For this review, take the finished solid that the model builds, in its own axes (mm). Face numbers are marked on the shaded views. A direction names the side the tool comes from. Round coordinates to 2 decimals unless told otherwise and drop trailing zeros. Order: outer loops, then holes, each group sorted by start corner. A loop starts at its lowest first (then second) coordinate and runs counter-clockwise, first axis right, second up. Notation, with made-up numbers: M -20,-14 L -12,-14 A15 cw -12,3 Z; hole C -15,-13 d6. An arc over 180 degrees is marked long. Answer in a Markdown table with one row per item. Add a question column.
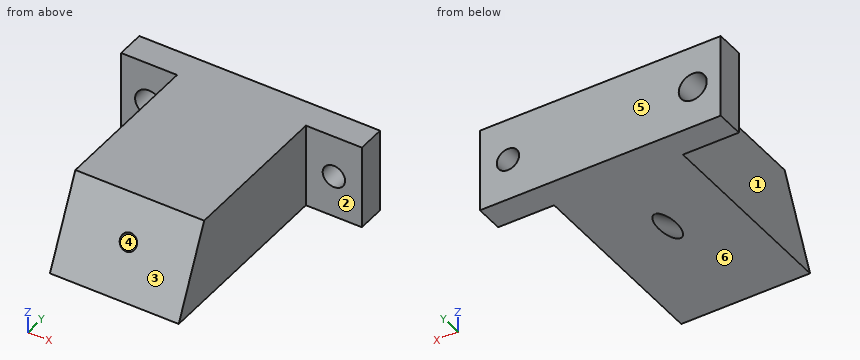
```python
from build123d import *

# Parameters (mm, degrees)
SKETCH1_W           = 23
SKETCH1_H           = 15
BOSS_EXTRUDE1_DEPTH = 40
CUT_EXTRUDE1_DEPTH  = 40
SKETCH3_R           = 1.5
CUT_EXTRUDE2_DEPTH  = 36
SKETCH4_W           = 15
SKETCH4_H           = 5
BOSS_EXTRUDE2_DEPTH = 10
SKETCH5_W           = 15
SKETCH5_H           = 5
BOSS_EXTRUDE3_DEPTH = 10
SKETCH6_R           = 2.5
SKETCH6_R_2         = 2
CUT_EXTRUDE3_DEPTH  = 10


with BuildPart() as part:
    # Sketch1 → Boss-Extrude1 (new body)
    with BuildSketch(Plane(origin=(0, 0, 0), x_dir=(1, 0, 0), z_dir=(0, 1, 0))):
        with Locations((-65.404761905, 8.571428571)):
            Rectangle(SKETCH1_W, SKETCH1_H)
    extrude(amount=BOSS_EXTRUDE1_DEPTH)

    # Sketch2 → Cut-Extrude1 (cut)
    with BuildSketch(Plane(origin=(-53.904761905, 0, 0), x_dir=(0, 0, -1), z_dir=(1, 0, 0))):
        Polygon((16.071428571, 0), (1.071428571, 0), (1.071428571, 6.994614872), align=None)
    extrude(amount=-CUT_EXTRUDE1_DEPTH, mode=Mode.SUBTRACT)

    # Sketch3 → Cut-Extrude2 (cut)
    with BuildSketch(Plane(origin=(0, 6.155714275, -2.870456708), x_dir=(1, 0, 0), z_dir=(0, -0.9063077870366528, 0.4226182617406934))):
        with Locations(Location((-65.378595466, -5.514992079, 0), (0, 0, 270))):
            Circle(SKETCH3_R)
    extrude(amount=-CUT_EXTRUDE2_DEPTH, mode=Mode.SUBTRACT)

    # Sketch4 → Boss-Extrude2 (add)
    with BuildSketch(Plane(origin=(-53.904761905, 0, 0), x_dir=(0, 0, -1), z_dir=(1, 0, 0))):
        with Locations((8.571428571, 37.5)):
            Rectangle(SKETCH4_W, SKETCH4_H)
    extrude(amount=BOSS_EXTRUDE2_DEPTH)

    # Sketch5 → Boss-Extrude3 (add)
    with BuildSketch(Plane.ZY.offset(76.904761905)):
        with Locations((-8.571428571, 37.5)):
            Rectangle(SKETCH5_W, SKETCH5_H)
    extrude(amount=BOSS_EXTRUDE3_DEPTH)

    # Sketch6 → Cut-Extrude3 (cut)
    with BuildSketch(Plane.XZ.offset(-35)):
        with Locations(Location((-81.904761905, -8.571428571, 0), (0, 0, 270))):
            Circle(SKETCH6_R)
        with Locations(Location((-48.904761905, -8.571428571, 0), (0, 0, 270))):
            Circle(SKETCH6_R_2)
    extrude(amount=-CUT_EXTRUDE3_DEPTH, mode=Mode.SUBTRACT)


solid = part.part
```
1. Consider section D-D on y = 30. Write out the cut boundary in (x, z), plus the area to 3 significant figures.
2. For the marked faces 1, 2 and 3, list the 3-axis set-ups (+Z, -Z, +X, -X, +Y, -Y) from which the entire face can be reached by the end or side of a thin tool; tool diameter is ignored.
3. Consider section B-B on x = -72. Write out the cut boundary in (y, z).
4. To check wall thickness, follow probe 1 along Y at (x, z) = (-83, -11); probe 2 along X at (y, z) = (20.5, -11); probe 3 along X at (y, z) = (7, -10.25). State the ranges of each line that lie inside material, in increasing order. Write a range as [from, to].
5. Consider section A-A on z = -9.75. State how many separate pieces and enclosed holes the cut face has, plus the area to 3 significant figures.
6. The part is to be moulded in two halves that separate along Y. For the marked faces 4, 5 and 6, say which applies: pulls with the +Y half, pulls with the -Y half, needs draft (parallel to the pull), parting line crosses it, or undercut.
7. Clearance check with flat-ended pins moving along their axes: pin 1 Ø2 at (y, z) = (6, -8.5) entering from -X; pin 2 Ø5 at (y, z) = (26.5, -6) entering from +X; pin 3 Ø8 at (x, z) = (-51.5, -7) entering from -Y. State where each tip first meets the part, or that it passes through.
Solved:
| question | item | result |
|---|---|---|
| 1 | outline | M -76.9,-16.07 L -53.9,-16.07 L -53.9,-1.07 L -76.9,-1.07 Z |
| 1 | area | 345 mm^2 |
| 2 | face 1 | +Z, -Z, -X, -Y |
| 2 | face 2 | +Z, -Z, +X, -Y |
| 2 | face 3 | +Z, +X, -X, -Y |
| 3 | outline | M 0,-16.07 L 40,-16.07 L 40,-1.07 L 6.99,-1.07 Z |
| 4 | probe 1 | y = [35, 40] |
| 4 | probe 2 | x = [-76.9, -53.9] |
| 4 | probe 3 | x = [-76.9, -66.64], [-64.12, -53.9] |
| 5 | separate pieces | 3 |
| 5 | enclosed holes | 1 |
| 5 | area | 897 mm^2 |
| 6 | face 4 | undercut |
| 6 | face 5 | pulls with the +Y half |
| 6 | face 6 | needs draft |
| 7 | pin 1 | stops at x = -76.9 |
| 7 | pin 2 | stops at x = -53.9 |
| 7 | pin 3 | stops at y = 2.74 |
